```python
from build123d import *

# Parameters (mm, degrees)
SKETCH2_W                        = 60
SKETCH2_H                        = 60
BOSS_EXTRUDE1_DEPTH              = 10
SKETCH7_W                        = 28
SKETCH7_H                        = 16
CUT_EXTRUDE2_DEPTH               = 44.588989435
FILLET2_R                        = 2
CBORE_FOR_M2_5_SHCS2_D           = 3.1
CBORE_FOR_M2_5_SHCS2_CBORE_D     = 5.5
CBORE_FOR_M2_5_SHCS2_CBORE_DEPTH = 2.5
MOVE_FACE1_BY                    = 3.5
MOVE_FACE1_2_BY                  = 3.5
MOVE_FACE1_3_BY                  = 3.5
MOVE_FACE1_4_BY                  = 3.5
SKETCH11_W                       = 10
SKETCH11_H                       = 5
BOSS_EXTRUDE2_DEPTH              = 60
SKETCH12_W                       = 20
SKETCH12_H                       = 60
BOSS_EXTRUDE3_DEPTH              = 10
CBORE_FOR_M4_SHCS1_D             = 4.8
CBORE_FOR_M4_SHCS1_CBORE_D       = 8
CBORE_FOR_M4_SHCS1_CBORE_DEPTH   = 4
FILLET5_R                        = 2


with BuildPart() as part:
    # Sketch2 → Boss-Extrude1 (new body)
    with BuildSketch(Plane(origin=(0, 0, 0), x_dir=(1, 0, 0), z_dir=(0, 1, 0))):
        Rectangle(SKETCH2_W, SKETCH2_H)
    extrude(amount=BOSS_EXTRUDE1_DEPTH)

    # Sketch7 → Cut-Extrude2 (cut, through all)
    with BuildSketch(Plane(origin=(0, 10, 0), x_dir=(1, 0, 0), z_dir=(0, 1, 0))):
        Rectangle(SKETCH7_W, SKETCH7_H)
    extrude(amount=-CUT_EXTRUDE2_DEPTH, mode=Mode.SUBTRACT)

    # Fillet2
    fillet2_edges = [part.edges().sort_by_distance(p)[0] for p in [
        (-14, 5, 8),
        (-14, 5, -8),
        (14, 5, -8),
        (14, 5, 8),
    ]]
    fillet(fillet2_edges, radius=FILLET2_R)

    # CBORE for M2.5 SHCS2 (through all)
    with Locations(Plane(origin=(0, 0, 0), x_dir=(-1, 0, 0), z_dir=(0, -1, 0))):
        with Locations((11, -20), (-11, -20), (11, 20), (-11, 20)):
            CounterBoreHole(CBORE_FOR_M2_5_SHCS2_D / 2, CBORE_FOR_M2_5_SHCS2_CBORE_D / 2, CBORE_FOR_M2_5_SHCS2_CBORE_DEPTH)

    # Move Face1: a face moved inward by 3.5
    extrude(part.faces().sort_by_distance((11, 2.5, 22.2))[0], amount=MOVE_FACE1_BY, dir=(0, 1, 0), mode=Mode.SUBTRACT)

    # Move Face1 2: a face moved inward by 3.5
    extrude(part.faces().sort_by_distance((-11, 2.5, 22.2))[0], amount=MOVE_FACE1_2_BY, dir=(0, 1, 0), mode=Mode.SUBTRACT)

    # Move Face1 3: a face moved inward by 3.5
    extrude(part.faces().sort_by_distance((11, 2.5, -17.8))[0], amount=MOVE_FACE1_3_BY, dir=(0, 1, 0), mode=Mode.SUBTRACT)

    # Move Face1 4: a face moved inward by 3.5
    extrude(part.faces().sort_by_distance((-11, 2.5, -17.8))[0], amount=MOVE_FACE1_4_BY, dir=(0, 1, 0), mode=Mode.SUBTRACT)

    # Sketch11 → Boss-Extrude2 (add)
    with BuildSketch(Plane(origin=(0, 0, -30), x_dir=(-1, 0, 0), z_dir=(0, 0, -1))):
        with Locations((-25, -2.5)):
            Rectangle(SKETCH11_W, SKETCH11_H)
    boss_extrude2 = extrude(amount=-BOSS_EXTRUDE2_DEPTH)

    # Sketch12 → Boss-Extrude3 (add)
    with BuildSketch(Plane.XZ.offset(5)):
        with Locations((40, 0)):
            Rectangle(SKETCH12_W, SKETCH12_H)
    boss_extrude3 = extrude(amount=-BOSS_EXTRUDE3_DEPTH)

    # CBORE for M4 SHCS1 (through all)
    with Locations(Plane(origin=(0, 5, 0), x_dir=(1, 0, 0), z_dir=(0, 1, 0))):
        with Locations((40, 20), (40, -20)):
            cbore_for_m4_shcs1 = CounterBoreHole(CBORE_FOR_M4_SHCS1_D / 2, CBORE_FOR_M4_SHCS1_CBORE_D / 2, CBORE_FOR_M4_SHCS1_CBORE_DEPTH)

    # Mirror1: Boss-Extrude2, Boss-Extrude3, CBORE for M4 SHCS1 across plane
    add(boss_extrude2.mirror(Plane(origin=(0, 0, 0), x_dir=(0, 0, 1), z_dir=(1, 0, 0))))
    add(boss_extrude3.mirror(Plane(origin=(0, 0, 0), x_dir=(0, 0, 1), z_dir=(1, 0, 0))))
    add(cbore_for_m4_shcs1.mirror(Plane(origin=(0, 0, 0), x_dir=(0, 0, 1), z_dir=(1, 0, 0))), mode=Mode.SUBTRACT)

    # Fillet5
    fillet5_edges = [part.edges().sort_by_distance(p)[0] for p in [
        (50, 5, 0),
        (30, 5, 0),
        (30, 10, 0),
        (-20, 0, 0),
        (-20, -5, 0),
        (-30, 5, 0),
        (-50, 5, 0),
        (-30, 10, 0),
        (20, 0, 0),
        (20, -5, 0),
    ]]
    fillet(fillet5_edges, radius=FILLET5_R)


solid = part.part
```
Can you work these out from the model? Positions are in its coordinate system, mm. A direction names the side the tool comes from. Round coordinates to 2 decimals unless told otherwise and drop trailing zeros. Loops run counter-clockwise (first coordinate to the right, second up) from the corner with the lowest first, then second, coordinate; pieces in that order, holes last. Notation, with made-up numbers: M 37,52 L 78,52 A24 cw 78,82 Z; hole C -16.75,-28.75 d8. An arc over 180 degrees is marked long. Write item = value, one per line. Start each with the question number.
(1) If we mould it in two halves opening along Z, with no side actions, what happens to faces 1 (the face through (-49.43, 4.4, 0.42)), 2 (the face through (13.4, 4.93, 7.43)), 3 (the face through (42, 1, -18))? For each: released by +Z, released by -Z, zero draft, split by the parting line, or undercut.
(2) I'm going to push flat-ended pins straight in: P1, Ø3.5, axis at x = 11, z = -20, coming from the -Y side; P2, Ø0.8, axis at y = 7.5, z = -5, coming from the -X side; P3, Ø9, axis at x = 40, z = -21, coming from the +Y side. Where does each tip first touch, or does it pass through?
(3) Suppose I cut it at D-D on y = -1. Write out the boundary of the cut face in (x, z).
(4) Suppose I cut it at B-B on x = 40. Write out the boundary of the cut face in (y, z), plus the area to 3 significant figures.
(5) I need wall thicknesses on line 1 along Z through (x, y) = (40, 3.95); line 2 along Z through (x, y) = (-11, 4.75); line 3 along Z through (x, y) = (40, -2.75). Which ranges of each line are inside material? Lowest first, please.
(6) Which directions (+Z, -Z, +X, -X, +Y, -Y) give clear straight access to the entire face, cutting with the end or side of a thin tool? Please do faces 4 (the face through (19.4, -0.57, 0.42)), 5 (the face through (-13.4, 4.93, -7.43)), 6 (the face through (40, 5, 0)), 7 (the face through (11, 6, 22)), 8 (the face through (37.05, 3.03, 17.3)).
(7) Suppose I cut it at C-C on z = -5. Write out the boundary of the cut face in (x, y), plus the area to 3 significant figures.
(8) Suppose I cut it at A-A on x = 1. Write out the boundary of the cut face in (y, z).
Answer block:
q1.face_1 = zero draft
q1.face_2 = undercut
q1.face_3 = undercut
q2.P1 = 6
q2.P2 = -30
q2.P3 = 5
q3.outline = M -50,-30 L -19.73,-30 L -19.73,30 L -50,30 Z; M 19.73,-30 L 50,-30 L 50,30 L 19.73,30 Z; hole C -40,-20 d4.8; hole C -40,20 d4.8; hole C 40,-20 d4.8; hole C 40,20 d4.8
q4.outline = M -5,-30 L 5,-30 L 5,-24 L 1,-24 L 1,-22.4 L -5,-22.4 Z; M -5,-17.6 L 1,-17.6 L 1,-16 L 5,-16 L 5,16 L 1,16 L 1,17.6 L -5,17.6 Z; M -5,22.4 L 1,22.4 L 1,24 L 5,24 L 5,30 L -5,30 Z
q4.area = 478 mm²
q5.line_1 = -30 to -24, -16 to 16, 24 to 30
q5.line_2 = -30 to -22.75, -17.25 to -8, 8 to 17.25, 22.75 to 30
q5.line_3 = -30 to -22.4, -17.6 to 17.6, 22.4 to 30
q6.face_4 = +Z, -Z, -Y
q6.face_5 = +Y, -Y
q6.face_6 = +Z, -Z, +X, +Y
q6.face_7 = -Y
q6.face_8 = +Y
q7.outline = M -50,-5 L -22,-5 A2 ccw -20,-3 L -20,-2 A2 cw -18,0 L -14,0 L -14,10 L -28,10 A2 ccw -30,8 L -30,7 A2 cw -32,5 L -48,5 A2 ccw -50,3 Z; M 14,0 L 18,0 A2 cw 20,-2 L 20,-3 A2 ccw 22,-5 L 50,-5 L 50,3 A2 ccw 48,5 L 32,5 A2 cw 30,7 L 30,8 A2 ccw 28,10 L 14,10 Z
q7.area = 818 mm²
q8.outline = M 0,-30 L 10,-30 L 10,-8 L 0,-8 Z; M 0,8 L 10,8 L 10,30 L 0,30 Z
